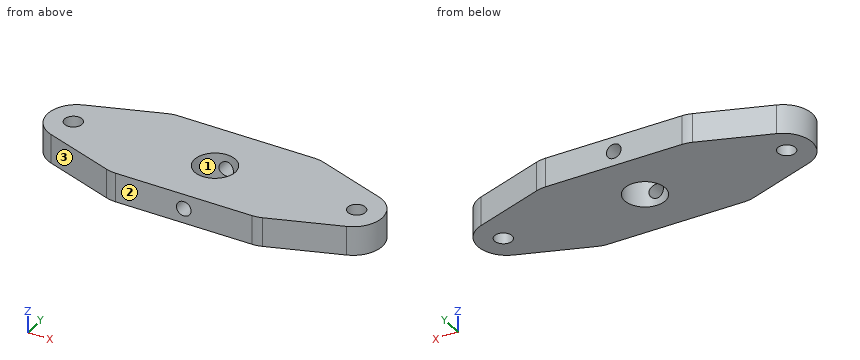
Autodesk Fusion 360 part; units mm, degrees
sketch "Main" plane through (0, 0, 0) normal (0, 0, 1) x (1, 0, 0)
  line L0 (-7.5, 5.5) -> (7.5, 5.5)
  line L1 (7.5, 5.5) -> (17.5, 2)
  line L2 (17.5, 2) -> (17.5, -2)
  line L3 (17.5, -2) -> (7.5, -5.5)
  line L4 (7.5, -5.5) -> (-7.5, -5.5)
  line L5 (-7.5, -5.5) -> (-17.5, -2)
  line L6 (-17.5, -2) -> (-17.5, 2)
  line L7 (-17.5, 2) -> (-7.5, 5.5)
  circle A0 centre (0, 0) radius 2.1
  dimension "d1" = 4.2
  dimension "d2" = 15
  dimension "d3" = 15
  dimension "d4" = 7.5
  dimension "d5" = 5.5
  dimension "d6" = 5.5
  dimension "d7" = 10
  dimension "d8" = 10
  dimension "d9" = 4
  dimension "d10" = 4
  dimension "d11" = 3.5
extrude "Extrude1" add sketch "Main" along normal blind 3
sketch "Face holes" plane through (0, 0, 3) normal (0, 0, 1) x (-1, 0, 0)
  circle A0 centre (0, 0) radius 2.1
  line L0 (17.5, -2) -> (17.5, 2)
  line L1 (17.5, 2) -> (7.5, 5.5)
  line L2 (7.5, 5.5) -> (-7.5, 5.5)
  line L3 (-7.5, 5.5) -> (-17.5, 2)
  line L4 (-17.5, 2) -> (-17.5, -2)
  line L5 (-17.5, -2) -> (-7.5, -5.5)
  line L6 (-7.5, -5.5) -> (7.5, -5.5)
  line L7 (7.5, -5.5) -> (17.5, -2)
  circle A1 centre (14.5, 0) radius 0.9
  circle A2 centre (-14.5, 0) radius 0.9
  dimension "d14" = 1.8
  dimension "d15" = 1.8
  dimension "d16" = 29
  dimension "d18" = 14.5
extrude "Extrude2" cut sketch "Face holes" against normal blind 3 contours A1 | A2
fillet "Fillet1" radius 3 8 edges at (-17.5, -2, 1.5) (-7.5, -5.5, 1.5) (7.5, -5.5, 1.5) (17.5, -2, 1.5) (17.5, 2, 1.5) (7.5, 5.5, 1.5) (-7.5, 5.5, 1.5) (-17.5, 2, 1.5)
sketch "Hole Pin" plane through (0, -5.5, 0) normal (0, -1, 0) x (1, 0, 0)
  line L0 (6.9902, 0) -> (6.9902, 3)
  line L1 (6.9902, 3) -> (-6.9902, 3)
  line L2 (-6.9902, 3) -> (-6.9902, 0)
  line L3 (-6.9902, 0) -> (6.9902, 0)
  circle A0 centre (0, 1.5) radius 0.75
  dimension "d23" = 1.5
  dimension "d24" = 1.5
extrude "Extrude3" cut sketch "Hole Pin" against normal blind 17 contours A0
Input: part model. Units: mm. Frame: model coordinates. Face numbers are marked on the shaded views. Coordinates: 2 decimals unless noted, no trailing zeros. Loops run counter-clockwise (first coordinate to the right, second up) from the corner with the lowest first, then second, coordinate; pieces in that order, holes last.
Q1. Material intervals for line 1 (Z direction, x = 0, y = 2.8); line 2 (X direction, y = 0.25, z = 1.5); line 3 (X direction, y = -0.5, z = 2.4), sorted ascending.
Q2. Cut plane A-A (x = -14.5). Output: boundary loops of the cut face in (y, z), then the cut area to 3 significant figures.
Q3. Cut plane B-B (z = 1.5). Give the number of separate pieces and of enclosed holes in the cut face, then the cut area to 3 significant figures.
Q4. Draft query along X for the marked faces 1, 2 and 3. Return one class per face: +X half, -X half, draft (parallel to the pull), parting line (faces both ways), or undercut.
Q5. Cut plane C-C (y = -4). Output: boundary loops of the cut face in (x, z).
Working result:
1. line 1: z = 0 to 0.75, 2.25 to 3
1. line 2: x = -17.12 to -15.36, -13.64 to -2.09, 2.09 to 13.64, 15.36 to 17.12
1. line 3: x = -17.09 to -15.25, -13.75 to -2.04, 2.04 to 13.75, 15.25 to 17.09
2. outline: (-3.05, 0) - (-0.9, 0) - (-0.9, 3) - (-3.05, 3) - close; (0.9, 0) - (3.05, 0) - (3.05, 3) - (0.9, 3) - close
2. area: 12.9 mm2
3. separate pieces: 2
3. enclosed holes: 2
3. area: 279 mm2
4. face 1: undercut
4. face 2: draft
4. face 3: -X half
5. outline: (-11.79, 0) - (11.79, 0) - (11.79, 3) - (-11.79, 3) - close; hole circle Ø1.5 at (0, 1.5)
